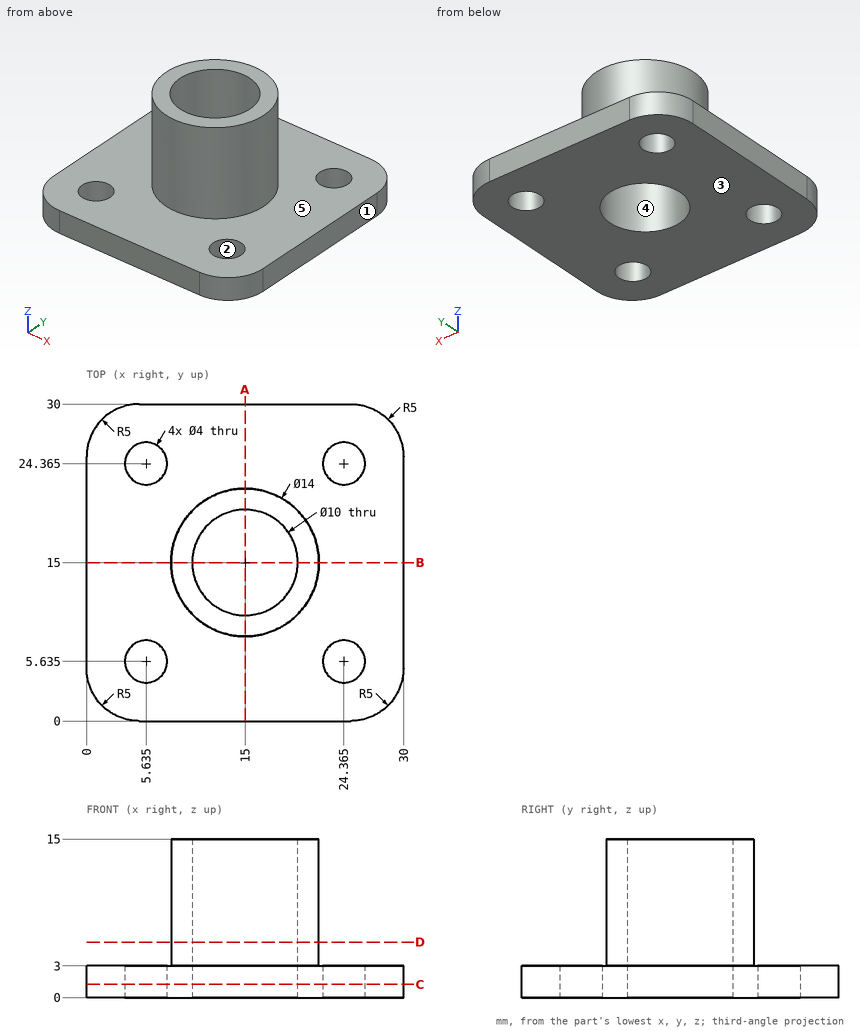
Print and shaded views of the part. All mm, measured from the part's lowest x, y and z. A direction names the side the tool comes from. Give positions to 0.01 mm unless a question says otherwise; leave off trailing zeros. Loops run counter-clockwise (first coordinate to the right, second up) from the corner with the lowest first, then second, coordinate; pieces in that order, holes last. Notation, with made-up numbers: (48, 6) - (79, 6) arc R15 ccw to (79, 18) - close; hole circle Ø1 at (-20, -37). An arc over 180 degrees is marked (long way). One line per item, written item: value. Start each with the question number.
1. Which spindle directions (+Z, -Z, +X, -X, +Y, -Y) get a long thin tool onto all of the face, cutting with end or side? Do the marked faces 4 and 5. Say none if no direction does.
2. Pin check, flat tips, straight feed: pin 1 (6.5 mm diameter, centred on x = 24.36, y = 24.36, fed in from +Z); pin 2 (3 mm diameter, centred on x = 9.5, z = 12.5, fed in from -Y) (1 decimal); pin 3 (8 mm diameter, centred on x = 15, y = 15, fed in from -Z); pin 4 (1.5 mm diameter, centred on y = 18.5, z = 10, fed in from +X). Stop position of each tip, or through.
3. Probe L1, parallel to Y at x = 15.25, z = 6.5 (1 decimal); L2, parallel to Y at x = 6.5, z = 2; L3, parallel to Z at x = 23.75, y = 28.25. List the from-to ranges inside material, lowest first. Write a range as from..to.
4. Slice it at D-D (z = 5.25). List the corners of the cut face in (x, y).
5. Slice it at A-A (x = 15). List the corners of the cut face in (y, z), plus the area to 3 significant figures.
6. Slice it at C-C (z = 1.25). List the corners of the cut face in (x, y) (1 decimal).
7. Pull direction X, two halves, no side cores. Call the marked faces 1, 2 and 3: pulls with the +X half, pulls with the -X half, needs draft (parallel to the pull), parting line crosses it, or undercut.
Solution:
1. face 4: +Z, -Z
1. face 5: +Z
2. pin 1: stops at z = 3
2. pin 2: stops at y = 9.3
2. pin 3: passes through
2. pin 4: stops at x = 21.44
3. L1: y = 8..10, 20..22
3. L2: y = 0..3.83, 7.44..22.56, 26.17..30
3. L3: z = 0..3
4. outline: circle Ø14 at (15, 15); hole circle Ø10 at (15, 15)
5. outline: (0, 0) - (10, 0) - (10, 15) - (8, 15) - (8, 3) - (0, 3) - close; (20, 0) - (30, 0) - (30, 3) - (22, 3) - (22, 15) - (20, 15) - close
5. area: 108 mm^2
6. outline: (0, 5) arc R5 ccw to (5, 0) - (25, 0) arc R5 ccw to (30, 5) - (30, 25) arc R5 ccw to (25, 30) - (5, 30) arc R5 ccw to (0, 25) - close; hole circle Ø4 at (5.6, 5.6); hole circle Ø4 at (5.6, 24.4); hole circle Ø10 at (15, 15); hole circle Ø4 at (24.4, 5.6); hole circle Ø4 at (24.4, 24.4)
7. face 1: pulls with the +X half
7. face 2: undercut
7. face 3: needs draft
